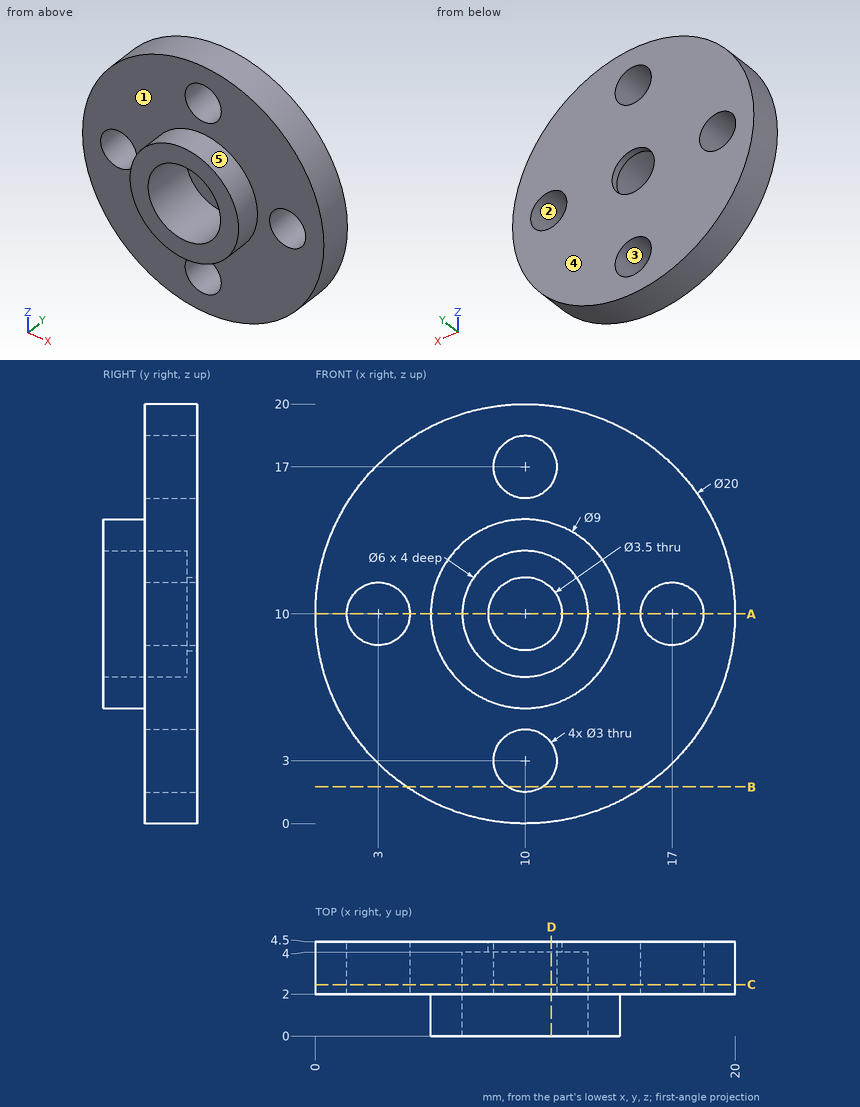
Check sheet for the drawn part. Datum: minimum x, y, z corner. Units: mm. A direction names the side the tool comes from. Round coordinates to 2 decimals unless told otherwise and drop trailing zeros. Write each loop counter-clockwise with the first axis right and the second up, starting at its lowest first coordinate (ties: lowest second). Pieces come first, ordered by that corner, then holes. Notation, with made-up numbers: (5.5, 53.25) -> (50.5, 53.25) arc R12 cw to (50.5, 63.25) -> close; hole circle Ø1 at (27, -3). An arc over 180 degrees is marked (long way). Write each question's results on one line, items separated by ' | '.
Q1. Sectioned sample at A-A, the plane z = 10. Record the boundary of the cut face in (x, y), and give its area (4 significant figures).
Derived:
outline: (0, 2) -> (1.5, 2) -> (1.5, 4.5) -> (0, 4.5) -> close; (4.5, 2) -> (5.5, 2) -> (5.5, 0) -> (7, 0) -> (7, 4) -> (8.25, 4) -> (8.25, 4.5) -> (4.5, 4.5) -> close; (11.75, 4) -> (13, 4) -> (13, 0) -> (14.5, 0) -> (14.5, 2) -> (15.5, 2) -> (15.5, 4.5) -> (11.75, 4.5) -> close; (18.5, 2) -> (20, 2) -> (20, 4.5) -> (18.5, 4.5) -> close | area: 27.25 mm²
Q2. Sectioned sample at D-D, the plane x = 11.25. Record the boundary of the cut face in (y, z).
Derived:
outline: (0, 5.68) -> (2, 5.68) -> (2, 3.83) -> (4.5, 3.83) -> (4.5, 8.78) -> (4, 8.78) -> (4, 7.27) -> (0, 7.27) -> close; (0, 12.73) -> (4, 12.73) -> (4, 11.22) -> (4.5, 11.22) -> (4.5, 16.17) -> (2, 16.17) -> (2, 14.32) -> (0, 14.32) -> close; (2, 0.08) -> (4.5, 0.08) -> (4.5, 2.17) -> (2, 2.17) -> close; (2, 17.83) -> (4.5, 17.83) -> (4.5, 19.92) -> (2, 19.92) -> close
Q3. Draft check along X on the marked faces 3, 4 and 5. Enter one of: released by +X, released by -X, zero draft, split by the parting line, or undercut.
Derived:
face 3: undercut | face 4: zero draft | face 5: split by the parting line
Q4. Go/stop test with flat-tipped pins: pin 1 Ø2 at (x, y) = (16.5, 1.5) entering from +Z; pin 2 Ø5 at (x, z) = (17.5, 5.5) entering from -Y; pin 3 Ø1 at (x, y) = (16.5, 0.5) entering from +Z; pin 4 Ø3 at (x, z) = (9, 10.5) entering from -Y. Record where each tip stops, or that it passes through.
Derived:
pin 1: stops at z = 18.26 | pin 2: stops at y = 2 | pin 3: passes through | pin 4: stops at y = 4
Q5. Access from +Z, -Z, +X, -X, +Y, -Y to the whole of each face (thin tool, end or side, straight path). Record for the marked faces 1 and 2.
Derived:
face 1: -Y | face 2: +Y, -Y
Q6. Sectioned sample at C-C, the plane y = 2.45. Record the boundary of the cut face in (x, z), and give its area (3 significant figures).
Derived:
outline: circle Ø20 at (10, 10); hole circle Ø3 at (3, 10); hole circle Ø6 at (10, 10); hole circle Ø3 at (10, 3); hole circle Ø3 at (10, 17); hole circle Ø3 at (17, 10) | area: 258 mm²
Q7. Sectioned sample at B-B, the plane z = 1.75. Record the boundary of the cut face in (x, y).
Derived:
outline: (4.35, 2) -> (9.17, 2) -> (9.17, 4.5) -> (4.35, 4.5) -> close; (10.83, 2) -> (15.65, 2) -> (15.65, 4.5) -> (10.83, 4.5) -> close
Q8. Thickness scan on probe 1 along X at (y, z) = (4.2, 10); probe 2 along Z at (x, y) = (10, 2.7). Record the ranges inside material, lowest first.
Derived:
probe 1: x = 0 to 1.5, 4.5 to 8.25, 11.75 to 15.5, 18.5 to 20 | probe 2: z = 0 to 1.5, 4.5 to 7, 13 to 15.5, 18.5 to 20
